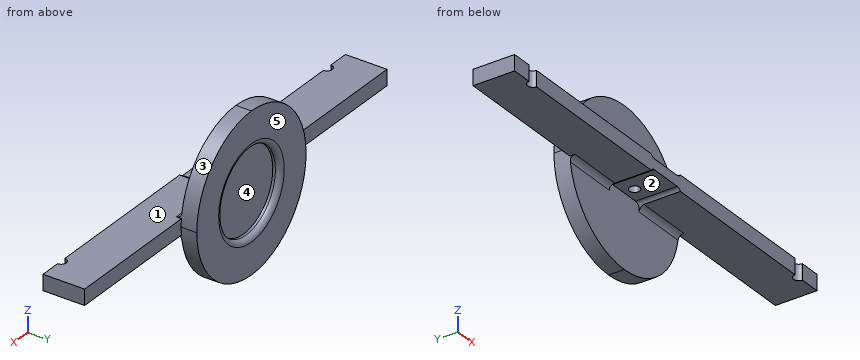
from build123d import *

# Parameters (mm, degrees)
SKETCH1_W                = 30
SKETCH1_H                = 30
BOSS_EXTRUDE1_DEPTH      = 3
BOSS_EXTRUDE2_DEPTH      = 1.5
BOSS_EXTRUDE2_DEPTH_BACK = 1.5
SKETCH2_W                = 83
SKETCH2_H                = 8
CUT_EXTRUDE1_DEPTH       = 46.370695388
SKETCH5_R                = 8
CUT_EXTRUDE2_DEPTH       = 1.5
FILLET1_R                = 1
SKETCH6_R                = 1
CUT_EXTRUDE3_DEPTH       = 10
CUT_EXTRUDE4_REACH       = 47.478
SKETCH9_W                = 8
SKETCH9_H                = 0.5
FILLET2_R                = 1
FILLET3_R                = 1
FILLET4_R                = 15


# Some blends are built 0.0001 mm under size
with BuildPart() as part:
    # Sketch1 → Boss-Extrude1 (new body)
    with BuildSketch(Plane(origin=(0, 0, 0), x_dir=(1, 0, 0), z_dir=(0, 1, 0))):
        Rectangle(SKETCH1_W, SKETCH1_H)
    extrude(amount=BOSS_EXTRUDE1_DEPTH)

    # Sketch2 → Boss-Extrude2 (add, two sides: drawn at the far end of the back side and taken through both)
    with BuildSketch(Plane.XY.offset(-BOSS_EXTRUDE2_DEPTH_BACK)):
        with Locations((0, -4)):
            Rectangle(SKETCH2_W, SKETCH2_H)
    extrude(amount=BOSS_EXTRUDE2_DEPTH + BOSS_EXTRUDE2_DEPTH_BACK)

    # Sketch4 → Cut-Extrude1 (cut, through all)
    with BuildSketch(Plane.XY.offset(1.5)):
        with BuildLine():
            ThreePointArc((-35.5, -8), (-36.5, -7), (-37.5, -8))
            Line((-37.5, -8), (-35.5, -8))
        make_face()
        with BuildLine():
            ThreePointArc((37.5, -8), (36.5, -7), (35.5, -8))
            Line((35.5, -8), (37.5, -8))
        make_face()
    extrude(amount=-CUT_EXTRUDE1_DEPTH, mode=Mode.SUBTRACT)

    # Sketch5 → Cut-Extrude2 (cut)
    with BuildSketch(Plane(origin=(0, 3, 0), x_dir=(1, 0, 0), z_dir=(0, 1, 0))):
        with Locations(Location((0, 0, 0), (0, 0, 270))):
            Circle(SKETCH5_R)
    extrude(amount=-CUT_EXTRUDE2_DEPTH, mode=Mode.SUBTRACT)

    # Fillet1
    fillet1_edges = [part.edges().sort_by_distance(p)[0] for p in [
        (0, 3, -8),
    ]]
    fillet(fillet1_edges, radius=FILLET1_R)

    # Sketch6 → Cut-Extrude3 (cut)
    with BuildSketch(Plane.XY.offset(1.5)):
        with Locations((0, -2)):
            Circle(SKETCH6_R)
    extrude(amount=-CUT_EXTRUDE3_DEPTH, mode=Mode.SUBTRACT)

    # Cut-Extrude4: up to this face of the body (flat: up to its plane)
    cut_extrude4_end = Plane(part.part.faces().sort_by_distance((0, 0, 8.25))[0])
    # Sketch9 → Cut-Extrude4 (cut, up to the picked face)
    with BuildSketch(Plane.XZ.offset(8), mode=Mode.PRIVATE) as cut_extrude4_sk1:
        with Locations((0, -1.25)):
            Rectangle(SKETCH9_W, SKETCH9_H)
    cut_extrude4_tool1 = split(extrude(cut_extrude4_sk1.sketch, amount=-CUT_EXTRUDE4_REACH, mode=Mode.PRIVATE), bisect_by=cut_extrude4_end, keep=Keep.BOTH, mode=Mode.PRIVATE)
    # Sketch9 → Cut-Extrude4 (cut, up to the picked face)
    with BuildSketch(Plane.XZ.offset(8), mode=Mode.PRIVATE) as cut_extrude4_sk2:
        with Locations((0, 1.25)):
            Rectangle(SKETCH9_W, SKETCH9_H)
    cut_extrude4_tool2 = split(extrude(cut_extrude4_sk2.sketch, amount=-CUT_EXTRUDE4_REACH, mode=Mode.PRIVATE), bisect_by=cut_extrude4_end, keep=Keep.BOTH, mode=Mode.PRIVATE)
    add(cut_extrude4_tool1.solids().sort_by(Axis((0, -8, -1.25), (0, 1, 0)))[0], mode=Mode.SUBTRACT)
    add(cut_extrude4_tool2.solids().sort_by(Axis((0, -8, 1.25), (0, 1, 0)))[0], mode=Mode.SUBTRACT)

    # Fillet2
    # the kernel refuses this fillet: 1 mm, written as the material it adds along each edge
    with BuildSketch(Plane(origin=(-4, -8, -1), x_dir=(0, 0, -1), z_dir=(0, 1, 0))) as fillet2_piece_1_section:
        with BuildLine():
            CenterArc((1, -0.866025404), FILLET2_R, 120, 60)
            Line((0, -0.866025404), (0, 0))
            Line((0, 0), (0.5, 0))
        make_face()
    fillet2_piece_1 = extrude(amount=10.165063509, mode=Mode.PRIVATE)
    fillet2_piece_1 = split(fillet2_piece_1, bisect_by=Plane(origin=(-3.634974596, 1.5, -1.132242545), z_dir=(0, -1, 0)), keep=Keep.TOP, mode=Mode.PRIVATE)
    add(fillet2_piece_1)
    with BuildSketch(Plane(origin=(4, -8, -1), x_dir=(0, 0, -1), z_dir=(0, 1, 0))) as fillet2_piece_2_section:
        with BuildLine():
            CenterArc((1, 0.866025404), FILLET2_R, 180, 60)
            Line((0, 0.866025404), (0, 0))
            Line((0, 0), (0.5, 0))
        make_face()
    fillet2_piece_2 = extrude(amount=10.165063509, mode=Mode.PRIVATE)
    fillet2_piece_2 = split(fillet2_piece_2, bisect_by=Plane(origin=(3.634974596, 1.5, -1.132242545), z_dir=(0, -1, 0)), keep=Keep.TOP, mode=Mode.PRIVATE)
    add(fillet2_piece_2)
    with BuildSketch(Plane(origin=(-4, -8, 1), x_dir=(0, 0, 1), z_dir=(0, 1, 0))) as fillet2_piece_3_section:
        with BuildLine():
            CenterArc((1, 0.866025404), FILLET2_R, 180, 60)
            Line((0, 0.866025404), (0, 0))
            Line((0, 0), (0.5, 0))
        make_face()
    fillet2_piece_3 = extrude(amount=10.165063509, mode=Mode.PRIVATE)
    fillet2_piece_3 = split(fillet2_piece_3, bisect_by=Plane(origin=(-3.634974596, 1.5, 1.132242545), z_dir=(0, -1, 0)), keep=Keep.TOP, mode=Mode.PRIVATE)
    add(fillet2_piece_3)
    with BuildSketch(Plane(origin=(4, -8, 1), x_dir=(0, 0, 1), z_dir=(0, 1, 0))) as fillet2_piece_4_section:
        with BuildLine():
            CenterArc((1, -0.866025404), FILLET2_R, 120, 60)
            Line((0, -0.866025404), (0, 0))
            Line((0, 0), (0.5, 0))
        make_face()
    fillet2_piece_4 = extrude(amount=10.165063509, mode=Mode.PRIVATE)
    fillet2_piece_4 = split(fillet2_piece_4, bisect_by=Plane(origin=(3.634974596, 1.5, 1.132242545), z_dir=(0, -1, 0)), keep=Keep.TOP, mode=Mode.PRIVATE)
    add(fillet2_piece_4)

    # Fillet3
    fillet3_edges = [part.edges().sort_by_distance(p)[0] for p in [
        (9.5, 0, -1.5),
        (9.5, 0, 1.5),
        (-9.5, 0, 1.5),
        (-9.5, 0, -1.5),
    ]]
    fillet(fillet3_edges, radius=FILLET3_R)

    # Fillet4
    fillet4_edges = [part.edges().sort_by_distance(p)[0] for p in [
        (-15, 1.5, -15),
        (15, 1.5, -15),
        (15, 1.5, 15),
        (-15, 1.5, 15),
    ]]
    fillet(fillet4_edges, radius=FILLET4_R - 0.0001)  # a hair under: the kernel refuses the full size


solid = part.part
Input: part model. Units: mm. Frame: model coordinates. Face numbers are marked on the shaded views. A direction names the side the tool comes from. Round coordinates to 2 decimals unless told otherwise and drop trailing zeros. Write each loop counter-clockwise with the first axis right and the second up, starting at its lowest first coordinate (ties: lowest second). Pieces come first, ordered by that corner, then holes.
1) Reachability of the marked faces 4 and 5 from +Z, -Z, +X, -X, +Y, -Y: full face, straight path, thin tool, end or side. Return the list, or none.
2) Cut plane A-A (y = -2). Return the cut outline in (x, z).
3) Draft query along X for the marked faces 1, 2 and 3. Return one class per face: pulls with the +X half, pulls with the -X half, needs draft (parallel to the pull), parting line crosses it, or undercut.
4) Cut plane D-D (x = 27). Return the cut outline in (y, z).
5) Cut plane C-C (x = -36.5). Return the cut outline in (y, z).
6) Contact query for flat-ended pins moving along their axis: P1, Ø3.5, axis at x = -28.5, z = 0, coming from the +Y side; P2, Ø4, axis at x = 5, z = 7, coming from the -Y side; P3, Ø2, axis at x = -4.5, y = -3, coming from the +Z side. Output: stop coordinate, or through.
7) Ray query, L1, parallel to Y at x = 0, z = -0.55; L2, parallel to X at y = 1.75, z = 0; L3, parallel to Z at x = 22, y = -4. Return the intervals inside material, ascending.
8) Cut plane B-B (y = -5.5). Return the cut outline in (x, z), then the cut area to 3 significant figures.
Geometry says:
1. face 4: +Y
1. face 5: +Z, -Z, +X, -X, +Y
2. outline: (-41.5, -1.5) - (-4, -1.5) arc R1 cw to (-3.13, -1) - (-1, -1) - (-1, 1) - (-3.13, 1) arc R1 cw to (-4, 1.5) - (-41.5, 1.5) - close; (1, -1) - (3.13, -1) arc R1 cw to (4, -1.5) - (41.5, -1.5) - (41.5, 1.5) - (4, 1.5) arc R1 cw to (3.13, 1) - (1, 1) - close
3. face 1: needs draft
3. face 2: undercut
3. face 3: pulls with the +X half
4. outline: (-8, -1.5) - (0, -1.5) - (0, 1.5) - (-8, 1.5) - close
5. outline: (-7, -1.5) - (0, -1.5) - (0, 1.5) - (-7, 1.5) - close
6. P1: stops at y = 0
6. P2: stops at y = 0
6. P3: stops at z = 1.5
7. L1: y = -8 to -3, -1 to 1.5
7. L2: x = -15 to -8, 8 to 15
7. L3: z = -1.5 to 1.5
8. outline: (-41.5, -1.5) - (-4, -1.5) arc R1 cw to (-3.13, -1) - (3.13, -1) arc R1 cw to (4, -1.5) - (41.5, -1.5) - (41.5, 1.5) - (4, 1.5) arc R1 cw to (3.13, 1) - (-3.13, 1) arc R1 cw to (-4, 1.5) - (-41.5, 1.5) - close
8. area: 242 mm2
